```python
from build123d import *

# Parameters (mm, degrees)
SKETCH_W        = 60
SKETCH_H        = 60
SKETCH_W_2      = 54
SKETCH_H_2      = 54
PAD_DEPTH       = 140
SKETCH001_R     = 2.75
POCKET_DEPTH    = 3
SKETCH002_R     = 2.75
POCKET001_DEPTH = 3


with BuildPart() as part:
    # Sketch → Pad (new body)
    with BuildSketch(Plane.XY):
        Rectangle(SKETCH_W, SKETCH_H)
        Rectangle(SKETCH_W_2, SKETCH_H_2, mode=Mode.SUBTRACT)
    extrude(amount=PAD_DEPTH)

    # Sketch001 (on Face2 of Pad) → Pocket (cut)
    with BuildSketch(Plane.YZ.offset(30)):
        with Locations((-20, 130)):
            Circle(SKETCH001_R)
        with Locations((20, 130)):
            Circle(SKETCH001_R)
        with Locations((-20, 90)):
            Circle(SKETCH001_R)
        with Locations((20, 90)):
            Circle(SKETCH001_R)
        with Locations((-20, 50)):
            Circle(SKETCH001_R)
        with Locations((20, 50)):
            Circle(SKETCH001_R)
        with Locations((-20, 10)):
            Circle(SKETCH001_R)
        with Locations((20, 10)):
            Circle(SKETCH001_R)
    extrude(amount=-POCKET_DEPTH, mode=Mode.SUBTRACT)

    # Sketch002 (on Face2 of Pocket) → Pocket001 (cut)
    with BuildSketch(Plane(origin=(-30, 0, 0), x_dir=(0, -1, 0), z_dir=(-1, 0, 0))):
        with Locations((-20, 130)):
            Circle(SKETCH002_R)
        with Locations((20, 129.999984)):
            Circle(SKETCH002_R)
        with Locations((-20.000016, 90)):
            Circle(SKETCH002_R)
        with Locations((19.999984, 89.999984)):
            Circle(SKETCH002_R)
    extrude(amount=-POCKET001_DEPTH, mode=Mode.SUBTRACT)


solid = part.part
```
Verification items for the finished model (mm, model axes). A direction names the side the tool comes from. Round coordinates to 2 decimals unless told otherwise and drop trailing zeros. Order: outer loops, then holes, each group sorted by start corner. A loop starts at its lowest first (then second) coordinate and runs counter-clockwise, first axis right, second up.
1) Cross-section at C-C, the plane y = 20. Give the number of separate pieces and of enclosed holes in the cut face, plus the area to 3 significant figures.
Geometry says:
separate pieces: 8
enclosed holes: 0
area: 741 mm2
2) Depth check by flat-ended pin: pin 1 (6.5 mm diameter, centred on y = 20, z = 130, fed in from +X). Enter the tip coordinate at first touch or a pass-through.
Geometry says:
pin 1: stops at x = 30
3) Material ranges on line 1 (Z direction, x = 28.8, y = -20); line 2 (X direction, y = -1.5, z = 122.5), recorded low to high.
Geometry says:
line 1: z = 0 to 7.25, 12.75 to 47.25, 52.75 to 87.25, 92.75 to 127.25, 132.75 to 140
line 2: x = -30 to -27, 27 to 30
4) Draft check along Y on faces 1 (the flat face through (0, -30, 69)), 2 (the cylindrical face through (-28.521, 20.596, 127.315)), 3 (the flat face through (-2, -29, 140)). Enter one of: +Y half, -Y half, draft (parallel to the pull), parting line (faces both ways), or undercut.
Geometry says:
face 1: -Y half
face 2: undercut
face 3: draft
5) Cross-section at B-B, the plane z = 50. Record the cut outline in (x, y), plus the area to 3 significant figures.
Geometry says:
outline: (-30, -30) - (30, -30) - (30, -22.75) - (27, -22.75) - (27, -27) - (-27, -27) - (-27, 27) - (27, 27) - (27, 22.75) - (30, 22.75) - (30, 30) - (-30, 30) - close; (27, -17.25) - (30, -17.25) - (30, 17.25) - (27, 17.25) - close
area: 651 mm2
6) Cross-section at A-A, the plane x = -17. Record the cut outline in (y, z).
Geometry says:
outline: (-30, 0) - (-27, 0) - (-27, 140) - (-30, 140) - close; (27, 0) - (30, 0) - (30, 140) - (27, 140) - close
7) Tool access check on faces 4 (the flat face through (0, -27, 69)), 5 (the cylindrical face through (28.521, -20.596, 127.315)), 6 (the cylindrical face through (28.521, 19.642, 52.727)). Record the directions out of +Z, -Z, +X, -X, +Y, -Y that give a thin tool (end or side, any length) a straight path to the whole face; none if there is none.
Geometry says:
face 4: +Z, -Z
face 5: +X, -X
face 6: +X
